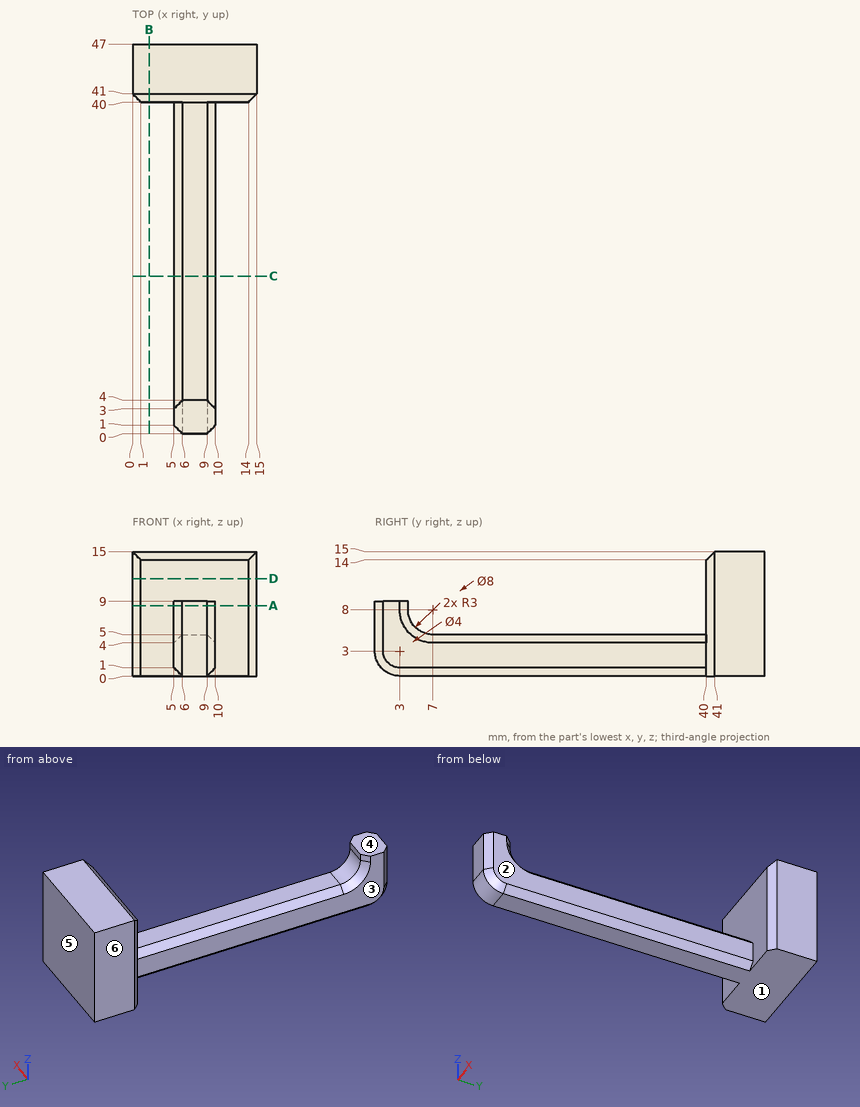
The figure shows three views and two pictorial views of one solid part (mm, origin at its lowest corner). Answer the questions. A direction names the side the tool comes from. Round coordinates to 2 decimals unless told otherwise and drop trailing zeros. Loops run counter-clockwise (first coordinate to the right, second up) from the corner with the lowest first, then second, coordinate; pieces in that order, holes last. Notation, with made-up numbers: (-27.5, 37.5) - (-22.5, 37.5) arc R26 cw to (-22.5, 72.5) - close; hole circle Ø10 at (-29.5, -16). An arc over 180 degrees is marked (long way). Use one line per item in the form item = value. Start each with the question number.
(1) Which of the six approach directions +Z, -Z, +X, -X, +Y, -Y give full straight-line access (tool end or side, diameter ignored) to the marked faces 1, 2, 3 and 4?
(2) Determine the mould class of the marked faces 5 and 6 for opening direction Y: +Y half, -Y half, draft (parallel to the pull), parting line (faces both ways), or undercut.
(3) Find section D-D on z = 11.75. Determine the outline of the cut face in (x, y).
(4) Find section B-B on x = 2. Determine the outline of the cut face in (y, z), and give its area (4 significant figures).
(5) Find section A-A on z = 8.5. Determine the outline of the cut face in (x, y).
(6) Flat-ended cylindrical pins translate along their axes: P1, Ø1.5, axis at x = 8, y = 31, coming from the +Z side; P2, Ø2, axis at x = 13, z = 8, coming from the -Y side; P3, Ø6.5, axis at y = 17, z = 5.5, coming from the +X side. Find the tip coordinate at first contact, or state that the pin passes through.
(7) Consider line 1 (Y direction, x = 4.5, z = 12.5); line 2 (Z direction, x = 7.25, y = 25); line 3 (Y direction, x = 7.75, z = 6). Determine where each line is inside the solid, lowest interval first.
(8) Find section C-C on y = 19. Determine the outline of the cut face in (x, z).
Answer list:
q1.face_1 = -Z, +X, -X, +Y, -Y
q1.face_2 = +Z, -Z, +X, -Y
q1.face_3 = +Z, -Z, -X, -Y
q1.face_4 = +Z, +X, -X, -Y
q2.face_5 = +Y half
q2.face_6 = draft
q3.outline = (0, 41) - (1, 40) - (14, 40) - (15, 41) - (15, 47) - (0, 47) - close
q4.outline = (40, 0) - (47, 0) - (47, 15) - (41, 15) - (40, 14) - close
q4.area = 104.5 mm^2
q5.outline = (0, 41) - (1, 40) - (14, 40) - (15, 41) - (15, 47) - (0, 47) - close; (5, 1) - (6, 0) - (9, 0) - (10, 1) - (10, 3) - (9, 4) - (6, 4) - (5, 3) - close
q6.P1 = 5
q6.P2 = 40
q6.P3 = 10
q7.line_1 = 40 to 47
q7.line_2 = 0 to 5
q7.line_3 = 0 to 4.76, 40 to 47
q8.outline = (5, 1) - (6, 0) - (9, 0) - (10, 1) - (10, 4) - (9, 5) - (6, 5) - (5, 4) - close
